Check sheet for the modelled part. Datum: model origin and axes. Units: mm. A direction names the side the tool comes from. Give positions to 0.01 mm unless a question says otherwise; leave off trailing zeros. Loops run counter-clockwise (first coordinate to the right, second up) from the corner with the lowest first, then second, coordinate; pieces in that order, holes last. Notation, with made-up numbers: (69.25, 18) -> (83.25, 18) arc R12 cw to (83.25, 22) -> close; hole circle Ø8 at (26.5, 24). An arc over 180 degrees is marked (long way). Answer as CSV lines item,"result". Start each with the question number.
(1) Section check B-B on x = 0. Enter the section's corners in (y, z), plus the area to 3 significant figures.
(2) Section check C-C on y = -13.5. Enter the section's corners in (x, z).
(3) Access from +Z, -Z, +X, -X, +Y, -Y to the whole of each face (thin tool, end or side, straight path). Record for faces 4 (the face through (2.5, -10, 7)), 5 (the face through (2.5, 11, 7)), 6 (the face through (-2.5, -10, 7)), 7 (the face through (-6, 0, 3)).
(4) Section check D-D on x = 13. Enter the section's corners in (y, z).
(5) Release check for a two-part mould opening along Y. For faces 1 (the face through (0, -17, 7)), 2 (the face through (-2.5, 10, 7)), 3 (the face through (-1.08, -4.88, 2.54)) record: pulls with the +Y half, pulls with the -Y half, needs draft (parallel to the pull), parting line crosses it, or undercut.
(6) Gauge pin test, flat ends, axial feed: pin 1 Ø8 at (x, y) = (-1.5, 1.5) entering from -Z; pin 2 Ø1 at (x, z) = (5, 7.5) entering from -Y; pin 3 Ø4 at (y, z) = (9.5, 8) entering from +X; pin 4 Ø5.5 at (y, z) = (-9.5, 8) entering from -X. Record the tip position at first contact, or that the pin passes through.
(7) Material ranges on line 1 (Y direction, x = 0, z = 1.35); line 2 (Z direction, x = 1, y = -12.5); line 3 (Y direction, x = 2, z = 1.5), recorded low to high. Write a range as from..to.
(8) Section check A-A on y = 0. Enter the section's corners in (x, z), plus the area to 3 significant figures.
from build123d import *

# Parameters (mm, degrees)
SWEEP_THIN1_PROFILE_R   = 6
SWEEP_THIN1_PROFILE_R_2 = 5
BOSS_EXTRUDE1_DEPTH     = 5


with BuildPart() as part:
    # Sweep-Thin1: sweep along a path in Sketch1
    with BuildLine(Plane.YZ) as sweep_thin1_path:
        Line((0, 0), (0, 5))
    # Sweep-Thin1 profile (on start of the path) → Sweep-Thin1 (sweep)
    with BuildSketch(Plane.XY):
        Circle(SWEEP_THIN1_PROFILE_R)
        Circle(SWEEP_THIN1_PROFILE_R_2, mode=Mode.SUBTRACT)
    sweep(path=sweep_thin1_path.line)

    # Sketch3 → Boss-Extrude1 (add)
    with BuildSketch(Plane.XY.offset(5)):
        with BuildLine():
            Line((-25, 2.5), (-2.5, 5.703923584))
            Line((-2.5, 5.703923584), (-2.5, 15.384581875))
            ThreePointArc((-2.5, 15.384581875), (0, 17.884581875), (2.5, 15.384581875))
            Line((2.5, 15.384581875), (2.5, 5.705628852))
            Line((2.5, 5.705628852), (25.349939608, 2.475387297))
            ThreePointArc((25.349939608, 2.475387297), (27.493839233, -0.175402049), (25, -2.5))
            Line((25, -2.5), (2.5, -5.703923584))
            Line((2.5, -5.703923584), (2.5, -14.498631066))
            ThreePointArc((2.5, -14.498631066), (0, -16.998631066), (-2.5, -14.498631066))
            Line((-2.5, -14.498631066), (-2.5, -5.703923584))
            Line((-2.5, -5.703923584), (-25, -2.5))
            ThreePointArc((-25, -2.5), (-27.5, 0), (-25, 2.5))
        make_face()
    extrude(amount=BOSS_EXTRUDE1_DEPTH)


solid = part.part
Working result:
1,outline,"(-17, 5) -> (-6, 5) -> (-6, 0) -> (-5, 0) -> (-5, 5) -> (5, 5) -> (5, 0) -> (6, 0) -> (6, 5) -> (17.88, 5) -> (17.88, 10) -> (-17, 10) -> close"
1,area,"184 mm^2"
2,outline,"(-2.5, 5) -> (2.5, 5) -> (2.5, 10) -> (-2.5, 10) -> close"
3,face 4,"+Z, -Z, +X, -Y"
3,face 5,"+Z, -Z, +X, +Y"
3,face 6,"+Z, -Z, -X, -Y"
3,face 7,"-Z"
4,outline,"(-4.21, 5) -> (4.22, 5) -> (4.22, 10) -> (-4.21, 10) -> close"
5,face 1,"pulls with the -Y half"
5,face 2,"needs draft"
5,face 3,"undercut"
6,pin 1,"stops at z = 0"
6,pin 2,"stops at y = -5.42"
6,pin 3,"stops at x = 2.5"
6,pin 4,"stops at x = -2.5"
7,line 1,"y = -6..-5, 5..6"
7,line 2,"z = 5..10"
7,line 3,"y = -5.66..-4.58, 4.58..5.66"
8,outline,"(-27.5, 5) -> (-6, 5) -> (-6, 0) -> (-5, 0) -> (-5, 5) -> (5, 5) -> (5, 0) -> (6, 0) -> (6, 5) -> (27.5, 5) -> (27.5, 10) -> (-27.5, 10) -> close"
8,area,"285 mm^2"
